```python
from build123d import *

# Parameters (mm, degrees)
F0_R          = 21.5
F1_DEPTH      = 57.15
F2_W          = 17.9596467465
F2_H          = 6.35
F2_W_2        = 17.1457676739
F3_DEPTH      = 21.501
F3_DEPTH_BACK = 21.501
F5_DEPTH      = 18.25
F6_W          = 28.575
F6_H          = 1.524
F7_DEPTH      = 6.35
F7_DEPTH_BACK = 23.368


with BuildPart() as f1:
    # F0 (on Top) → F1 (new body)
    with BuildSketch(Plane.XY):
        Circle(F0_R)
    extrude(amount=F1_DEPTH)

    # F2 (on Front) → F3 (cut, two sides)
    with BuildSketch(Plane.XZ) as f3_sk:
        with Locations((-18.1048233733, 3.175)):
            Rectangle(F2_W, F2_H)
        with Locations((17.6978838369, 3.175)):
            Rectangle(F2_W_2, F2_H)
    extrude(amount=-F3_DEPTH, mode=Mode.SUBTRACT)
    extrude(f3_sk.sketch, amount=F3_DEPTH_BACK, mode=Mode.SUBTRACT)

    # F4 (on face) → F5 (join, through all)
    with BuildSketch(Plane(origin=(-9.125, 0, 0), x_dir=(0, -1, 0), z_dir=(-1, 0, 0))):
        with BuildLine():
            Line((-21.5, 0), (-21.5, -2.7665854228))
            ThreePointArc((-21.5, -2.7665854228), (-30.4593629233, -32.216128711), (0.3193392569, -31.75))
            Line((0.3193392569, -31.75), (10.16, -31.75))
            Line((10.16, -31.75), (10.16, 0))
            Line((10.16, 0), (-19.4675210286, 0))
            Line((-19.4675210286, 0), (-21.5, 0))
        make_face()
    extrude(amount=-F5_DEPTH)

    # F6 (on face) → F7 (join, two sides)
    with BuildSketch(Plane(origin=(-9.125, 0, 0), x_dir=(0, -1, 0), z_dir=(-1, 0, 0))) as f7_sk:
        with Locations((-6.6675, 0.762)):
            Rectangle(F6_W, F6_H)
    extrude(amount=-F7_DEPTH)
    extrude(f7_sk.sketch, amount=F7_DEPTH_BACK)


solid = f1.part
```
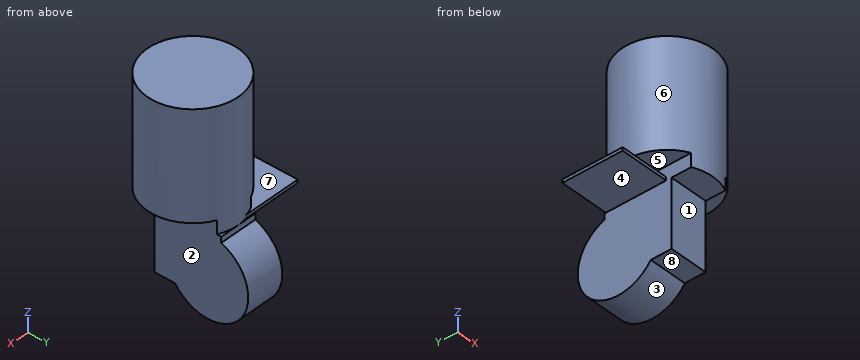
Geometry check sheet. Reference: the model listing, model coordinates, mm. Face numbers are marked on the shaded views. A direction names the side the tool comes from. Coordinates: 2 decimals unless noted, no trailing zeros. Write each loop counter-clockwise with the first axis right and the second up, starting at its lowest first coordinate (ties: lowest second). Pieces come first, ordered by that corner, then holes. Notation, with made-up numbers: (3, 58.25) -> (36, 58.25) arc R29 cw to (36, 91.25) -> close; hole circle Ø2 at (77.5, 89). An arc over 180 degrees is marked (long way). Use CSV: the item, a comma, the result in double quotes. Start each with the question number.
Item 1: Cross-section at D-D, the plane z = 44. Record the cut outline in (x, y), plus the area to 3 significant figures.
Item 2: Thickness scan on line 1 (Z direction, x = -14.5, y = -9.5); line 2 (Z direction, x = 0, y = -3); line 3 (Y direction, x = -6.5, z = -21). Record the ranges inside material, lowest first.
Item 3: Set-up check for the marked faces 1, 2, 3, 4 and 5: record each of +Z, -Z, +X, -X, +Y, -Y from which the full face is reachable in a straight line by a thin tool's end or side.
Item 4: Mould release check, pull along Z, two halves, no side actions. Record for the marked faces 6, 7 and 8: released by +Z, released by -Z, zero draft, split by the parting line, or undercut.
Item 5: Cross-section at C-C, the plane x = -24. Record the cut outline in (y, z) (3 decimals).
Item 6: Cross-section at B-B, the plane y = -12.5. Record the cut outline in (x, z) (3 decimals), plus the area to 3 significant figures.
Item 7: Depth check by flat-ended pin: pin 1 Ø0.8 at (x, z) = (-23, 0.5) entering from +Y (3 decimals); pin 2 Ø6 at (x, y) = (-17.5, 8.5) entering from -Z; pin 3 Ø10 at (y, z) = (8.5, 31.5) entering from +X; pin 4 Ø5 at (x, y) = (-6, 14) entering from -Z. Enter the tip coordinate at first touch or a pass-through.
Item 8: Cross-section at A-A, the plane x = -16.5. Record the cut outline in (y, z) (3 decimals), plus the area to 3 significant figures.
Answers:
1,outline,"circle Ø43 at (0, 0)"
1,area,"1,450 mm^2"
2,line 1,"6.35 to 57.15"
2,line 2,"-31.75 to 57.15"
2,line 3,"-10.16 to 34.29"
3,face 1,"-Z, +X, -X, -Y"
3,face 2,"-Z, +X, +Y, -Y"
3,face 3,"+X, -X"
3,face 4,"-Z, -X, +Y, -Y"
3,face 5,"-X, +Y, -Y"
4,face 6,"zero draft"
4,face 7,"undercut"
4,face 8,"released by -Z"
5,outline,"(-7.62, 0) -> (20.955, 0) -> (20.955, 1.524) -> (-7.62, 1.524) -> close"
6,outline,"(-17.493, 6.35) -> (-9.125, 6.35) -> (-9.125, 0) -> (9.125, 0) -> (9.125, 6.35) -> (17.493, 6.35) -> (17.493, 57.15) -> (-17.493, 57.15) -> close"
6,area,"1,890 mm^2"
7,pin 1,"y = 20.955"
7,pin 2,"z = 0"
7,pin 3,"x = 21.21"
7,pin 4,"z = -39.81"
8,outline,"(-13.784, 6.35) -> (13.784, 6.35) -> (13.784, 57.15) -> (-13.784, 57.15) -> close; (-7.62, 0) -> (20.955, 0) -> (20.955, 1.524) -> (-7.62, 1.524) -> close"
8,area,"1,440 mm^2"
